```python
from build123d import *

# Parameters (mm, degrees)
SKETCH5_W           = 40
SKETCH5_H           = 40
BOSS_EXTRUDE2_DEPTH = 2
CUT_EXTRUDE1_DEPTH  = 2
CUT_EXTRUDE4_DEPTH  = 2
CUT_EXTRUDE5_DEPTH  = 2
CUT_EXTRUDE6_DEPTH  = 2
CUT_EXTRUDE7_DEPTH  = 2
CUT_EXTRUDE8_DEPTH  = 2
SKETCH6_OUTSIDE_W   = 53.32
SKETCH6_OUTSIDE_H   = 53.32
SKETCH6_OUTSIDE_W_2 = 39.9
SKETCH6_OUTSIDE_H_2 = 39.9
CUT_EXTRUDE9_DEPTH  = 10


with BuildPart() as part:
    # Sketch5 → Boss-Extrude2 (new body)
    with BuildSketch(Plane.XY):
        Rectangle(SKETCH5_W, SKETCH5_H)
    extrude(amount=BOSS_EXTRUDE2_DEPTH)

    # Sketch4 → Cut-Extrude1 (cut)
    with BuildSketch(Plane.XY):
        Polygon((18, 16.585786438), (18, 10.414213562), (14.914213562, 13.5), align=None)
        Polygon((10.414213562, 18.056847711), (16.585786438, 18.056847711), (13.5, 14.971061274), align=None)
    extrude(amount=CUT_EXTRUDE1_DEPTH, mode=Mode.SUBTRACT)

    # Sketch4_5 → Cut-Extrude4 (cut)
    with BuildSketch(Plane.XY):
        Polygon((-13.5, -14.914213562), (-16.585786438, -18), (-10.414213562, -18), align=None)
        Polygon((-5.914213562, -13.5), (-9, -16.585786438), (-12.085786438, -13.5), (-9, -10.414213562), align=None)
        Polygon((-13.5, -5.914213562), (-10.414213562, -9), (-13.5, -12.085786438), (-16.585786438, -9), align=None)
        Polygon((-18, -16.585786438), (-18, -10.414213562), (-14.914213562, -13.5), align=None)
    extrude(amount=CUT_EXTRUDE4_DEPTH, mode=Mode.SUBTRACT)

    # Sketch4_6 → Cut-Extrude5 (cut)
    with BuildSketch(Plane.XY):
        Polygon((-1.414213562, -18), (-7.585786438, -18), (-4.5, -14.914213562), align=None)
        Polygon((3.085786438, -13.5), (0, -16.585786438), (-3.085786438, -13.5), (0, -10.414213562), align=None)
        Polygon((7.585786438, -18), (1.414213562, -18), (4.5, -14.914213562), align=None)
        Polygon((12.085786438, -13.5), (9, -16.585786438), (5.914213562, -13.5), (9, -10.414213562), align=None)
        Polygon((13.5, -14.914213562), (16.585786438, -18), (10.414213562, -18), align=None)
        Polygon((18, -10.414213562), (18, -16.585786438), (14.914213562, -13.5), align=None)
        Polygon((13.5, -5.914213562), (16.585786438, -9), (13.5, -12.085786438), (10.414213562, -9), align=None)
        Polygon((4.5, -5.914213562), (7.585786438, -9), (4.5, -12.085786438), (1.414213562, -9), align=None)
        Polygon((12.085786438, -4.5), (9, -7.585786438), (5.914213562, -4.5), (9, -1.414213562), align=None)
        Polygon((18, -1.414213562), (18, -7.585786438), (14.914213562, -4.5), align=None)
    extrude(amount=CUT_EXTRUDE5_DEPTH, mode=Mode.SUBTRACT)

    # Sketch4_7 → Cut-Extrude6 (cut)
    with BuildSketch(Plane.XY):
        Polygon((13.5, 3.085786438), (16.585786438, 0), (13.5, -3.085786438), (10.414213562, 0), align=None)
        Polygon((18, 7.585786438), (18, 1.414213562), (14.914213562, 4.5), align=None)
        Polygon((13.5, 12.085786438), (16.585786438, 9), (13.5, 5.914213562), (10.414213562, 9), align=None)
        Polygon((12.085786438, 4.5), (9, 1.414213562), (5.914213562, 4.5), (9, 7.585786438), align=None)
        Polygon((4.5, 12.085786438), (7.585786438, 9), (4.5, 5.914213562), (1.414213562, 9), align=None)
        Polygon((12.085786438, 13.5), (9, 10.414213562), (5.914213562, 13.5), (9, 16.585786438), align=None)
        Polygon((1.357365851, 18.056847711), (7.642634149, 18.056847711), (4.5, 14.914213562), align=None)
        Polygon((3.085786438, 13.5), (0, 10.414213562), (-3.085786438, 13.5), (0, 16.585786438), align=None)
        Polygon((3.085786438, 4.5), (0, 1.414213562), (-3.085786438, 4.5), (0, 7.585786438), align=None)
        Polygon((4.5, 3.085786438), (7.585786438, 0), (4.5, -3.085786438), (1.414213562, 0), align=None)
        Polygon((3.085786438, -4.5), (0, -7.585786438), (-3.085786438, -4.5), (0, -1.414213562), align=None)
        Polygon((-4.5, -5.914213562), (-1.414213562, -9), (-4.5, -12.085786438), (-7.585786438, -9), align=None)
    extrude(amount=CUT_EXTRUDE6_DEPTH, mode=Mode.SUBTRACT)

    # Sketch4_9 → Cut-Extrude7 (cut)
    with BuildSketch(Plane.XY):
        Polygon((-9, 1.414213562), (-12.085786438, 4.5), (-9, 7.585786438), (-5.914213562, 4.5), align=None)
        Polygon((-4.5, 3.085786438), (-1.414213562, 0), (-4.5, -3.085786438), (-7.585786438, 0), align=None)
        Polygon((-9, -7.585786438), (-12.085786438, -4.5), (-9, -1.414213562), (-5.914213562, -4.5), align=None)
        Polygon((-13.5, 3.085786438), (-10.414213562, 0), (-13.5, -3.085786438), (-16.585786438, 0), align=None)
        Polygon((-18, -7.585786438), (-18, -1.414213562), (-14.914213562, -4.5), align=None)
        Polygon((-18, 1.414213562), (-18, 7.585786438), (-14.914213562, 4.5), align=None)
    extrude(amount=CUT_EXTRUDE7_DEPTH, mode=Mode.SUBTRACT)

    # Sketch4_10 → Cut-Extrude8 (cut)
    with BuildSketch(Plane.XY):
        Polygon((-4.5, 12.085786438), (-1.414213562, 9), (-4.5, 5.914213562), (-7.585786438, 9), align=None)
        Polygon((-9, 10.414213562), (-12.085786438, 13.5), (-9, 16.585786438), (-5.914213562, 13.5), align=None)
        Polygon((-13.5, 12.085786438), (-10.414213562, 9), (-13.5, 5.914213562), (-16.585786438, 9), align=None)
        Polygon((-14.914213562, 13.5), (-18, 10.414213562), (-18, 16.585786438), align=None)
        Polygon((-10.357365851, 18.056847711), (-13.5, 14.914213562), (-16.642634149, 18.056847711), align=None)
        Polygon((-7.642634149, 18.056847711), (-1.357365851, 18.056847711), (-4.5, 14.914213562), align=None)
    extrude(amount=CUT_EXTRUDE8_DEPTH, mode=Mode.SUBTRACT)

    # Sketch6 outside → Cut-Extrude9 (cut)
    with BuildSketch(Plane(origin=(0, 0, 0), x_dir=(-1, 0, 0), z_dir=(0, 0, -1))):
        Rectangle(SKETCH6_OUTSIDE_W, SKETCH6_OUTSIDE_H)
        Rectangle(SKETCH6_OUTSIDE_W_2, SKETCH6_OUTSIDE_H_2, mode=Mode.SUBTRACT)
    extrude(amount=-CUT_EXTRUDE9_DEPTH, mode=Mode.SUBTRACT)


solid = part.part
```
Read the model definition and answer for the solid it produces. Units are mm, in the model's axes. Give positions to 0.01 mm unless a question says otherwise; leave off trailing zeros. Loops run counter-clockwise (first coordinate to the right, second up) from the corner with the lowest first, then second, coordinate; pieces in that order, holes last.
Item 1: The part is cut by section C-C (z = 1.6). Give the number of separate pieces and of enclosed holes in the cut face, and give its area (3 significant figures).
Item 2: Find the intervals of material crossed by line 1 along X through (y, z) = (-14, 0.6); line 2 along X through (y, z) = (-10, 0.65), in increasing order.
Item 3: The part is cut by section A-A (y = 14). Write down the section's boundary in (x, z), and give its area (3 significant figures).
Item 4: The part is cut by section B-B (x = -13). Write down the section's boundary in (y, z), and give its area (3 significant figures).
Item 5: This flat-tipped pin is pushed along its axis until it touches: pin 1 Ø1.5 at (x, y) = (1.5, 13.5) entering from -Z. Where does it stop, or does it pass through?
Item 6: The mould has two halves that part along X. Classify faces 1 (the flat face through (-7.479, -2.936, 0.986)), 2 (the flat face through (-2.936, 7.479, 0.986)): released by +X, released by -X, zero draft, split by the parting line, or undercut.
Taken from the geometry:
1. separate pieces: 1
1. enclosed holes: 40
1. area: 982 mm2
2. line 1: x = -19.95 to -18, -15.41 to -11.59, -6.41 to -2.59, 2.59 to 6.41, 11.59 to 15.41, 18 to 19.95
2. line 2: x = -19.95 to -15.59, -11.41 to -6.59, -2.41 to 2.41, 6.59 to 11.41, 15.59 to 19.95
3. outline: (-19.95, 0) - (-18, 0) - (-18, 2) - (-19.95, 2) - close; (-15.41, 0) - (-11.59, 0) - (-11.59, 2) - (-15.41, 2) - close; (-6.41, 0) - (-2.59, 0) - (-2.59, 2) - (-6.41, 2) - close; (2.59, 0) - (6.41, 0) - (6.41, 2) - (2.59, 2) - close; (11.59, 0) - (15.41, 0) - (15.41, 2) - (11.59, 2) - close; (18, 0) - (19.95, 0) - (19.95, 2) - (18, 2) - close
3. area: 38.4 mm2
4. outline: (-19.95, 0) - (-18, 0) - (-18, 2) - (-19.95, 2) - close; (-15.41, 0) - (-11.59, 0) - (-11.59, 2) - (-15.41, 2) - close; (-6.41, 0) - (-2.59, 0) - (-2.59, 2) - (-6.41, 2) - close; (2.59, 0) - (6.41, 0) - (6.41, 2) - (2.59, 2) - close; (11.59, 0) - (15.41, 0) - (15.41, 2) - (11.59, 2) - close; (18.06, 0) - (19.95, 0) - (19.95, 2) - (18.06, 2) - close
4. area: 38.3 mm2
5. pin 1: passes through
6. face 1: undercut
6. face 2: undercut
